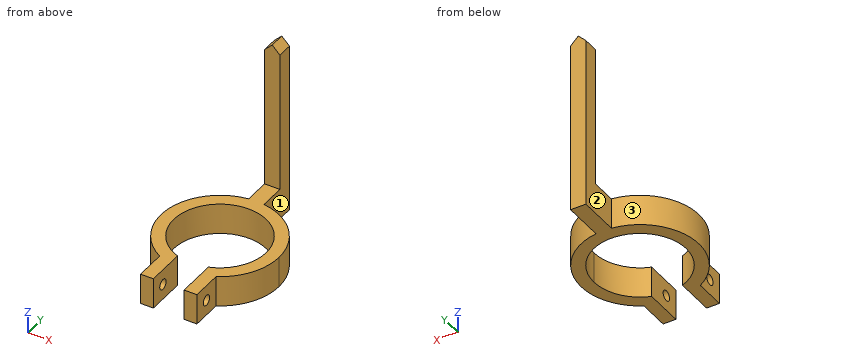
```python
from build123d import *

# Parameters (mm, degrees)
F1_DEPTH = 6
F2_W     = 3
F2_H     = 3
F3_DEPTH = 29
F5_D     = 2
F6_SIZE  = 1.49999


# Not quite as in the source:
# - a fillet or chamfer is up to 0.001 mm smaller than in the source, because OpenCascade refuses the exact size


with BuildPart() as f1:
    # F0 (on Top) → F1 (new body)
    with BuildSketch(Plane.XY):
        with BuildLine():
            ThreePointArc((-3, -8.4852813742), (-5.1961524227, 7.3484692283), (9, 0))
            ThreePointArc((9, 0), (7.3484692283, -5.1961524227), (3, -8.4852813742))
            Line((3, -8.4852813742), (3, -11.1018016556))
            ThreePointArc((3, -11.1018016556), (4.2794450198, -10.6740971666), (5.5, -10.0995049384))
            ThreePointArc((5.5, -10.0995049384), (9.8868599666, -5.8736700622), (11.5, 0))
            ThreePointArc((11.5, 0), (8.6458082329, 7.5828754441), (1.5, 11.401754251))
            ThreePointArc((1.5, 11.401754251), (0, 11.5), (-1.5, 11.401754251))
            ThreePointArc((-1.5, 11.401754251), (-11.3060177199, 2.103321972), (-5.5, -10.0995049384))
            ThreePointArc((-5.5, -10.0995049384), (-4.2794450198, -10.6740971666), (-3, -11.1018016556))
            Line((-3, -11.1018016556), (-3, -8.4852813742))
        make_face()
        with BuildLine():
            ThreePointArc((5.5, -10.0995049384), (4.2794450198, -10.6740971666), (3, -11.1018016556))
            Line((3, -11.1018016556), (3, -16.0995049384))
            Line((3, -16.0995049384), (5.5, -16.0995049384))
            Line((5.5, -16.0995049384), (5.5, -10.0995049384))
        make_face()
        with BuildLine():
            Line((-3, -16.0995049384), (-3, -11.1018016556))
            ThreePointArc((-3, -11.1018016556), (-4.2794450198, -10.6740971666), (-5.5, -10.0995049384))
            Line((-5.5, -10.0995049384), (-5.5, -16.0995049384))
            Line((-5.5, -16.0995049384), (-3, -16.0995049384))
        make_face()
        with BuildLine():
            Line((-1.5, 19.401754251), (-1.5, 11.401754251))
            ThreePointArc((-1.5, 11.401754251), (0, 11.5), (1.5, 11.401754251))
            Line((1.5, 11.401754251), (1.5, 19.401754251))
            Line((1.5, 19.401754251), (-1.5, 19.401754251))
        make_face()
    extrude(amount=F1_DEPTH)

    # F2 (on face) → F3 (join)
    with BuildSketch(Plane.XY.offset(6)):
        with Locations((0, 17.901754251)):
            Rectangle(F2_W, F2_H)
    extrude(amount=F3_DEPTH)

    # F5 (through all)
    with Locations(Plane(origin=(-5.5, 0, 0), x_dir=(0, -1, 0), z_dir=(-1, 0, 0))):
        with Locations((13.0995049384, 3)):
            Hole(F5_D / 2)

    # F6 (size 1.5 in the source; OpenCascade refuses exactly that, so slightly less here)
    f6_edges = [f1.edges().sort_by_distance(p)[0] for p in [
        (1.5, 17.901754, 35),
        (-1.5, 17.901754, 35),
    ]]
    chamfer(f6_edges, length=F6_SIZE)


solid = f1.part
```
The model under review builds one solid part; all positions refer to its coordinate system, in mm. Face numbers are marked on the shaded views. A direction names the side the tool comes from. Round coordinates to 2 decimals unless told otherwise and drop trailing zeros. Write each loop counter-clockwise with the first axis right and the second up, starting at its lowest first coordinate (ties: lowest second). Pieces come first, ordered by that corner, then holes.
(1) We need section A-A on z = 3. Give the boundary of the cut face in (x, y).
(2) Machinability: for the marked faces 1, 2 and 3, which of the approach directions +Z, -Z, +X, -X, +Y, -Y give a long, thin tool a straight path to every point of the face, cutting with its end or side? Answer none if there is none.
(3) We need section C-C on y = 2. Give the boundary of the cut face in (x, z).
(4) Insertion check: pin 1 (8 mm diameter, centred on x = -4.5, y = -10.5, fed in from -Z); pin 2 (6.5 mm diameter, centred on y = -12.5, z = 4, fed in from -X); pin 3 (10 mm diameter, centred on y = 14.5, z = 25.5, fed in from -X); pin 4 (2 mm diameter, centred on y = 16, z = 18.5, fed in from +X). Each pin has a flat end and moves straight along its axis. Give the tip position at first contact, or say it passes through.
(5) We need section B-B on x = 8.5. Give the boundary of the cut face in (y, z).
(6) Wall thickness on L1, parallel to Z at x = 9.75, y = 3.5; L2, parallel to Y at x = 0, z = 1.55; L3, parallel to X at y = 17.5, z = 18.5: over which ranges is each line inside the solid? List them lowest first.
Findings below:
1. outline: (-5.5, -16.1) - (-3, -16.1) - (-3, -14.1) - (-5.5, -14.1) - close; (-5.5, -12.1) - (-3, -12.1) - (-3, -8.49) arc R9 cw (long way) to (3, -8.49) - (3, -12.1) - (5.5, -12.1) - (5.5, -10.1) arc R11.5 ccw to (1.5, 11.4) - (1.5, 19.4) - (-1.5, 19.4) - (-1.5, 11.4) arc R11.5 ccw to (-5.5, -10.1) - close; (3, -16.1) - (5.5, -16.1) - (5.5, -14.1) - (3, -14.1) - close
2. face 1: +Z, -Z, +X, +Y
2. face 2: +Z, -Z, -X, +Y
2. face 3: +Z, -Z, -X
3. outline: (-11.32, 0) - (-8.77, 0) - (-8.77, 6) - (-11.32, 6) - close; (8.77, 0) - (11.32, 0) - (11.32, 6) - (8.77, 6) - close
4. pin 1: stops at z = 0
4. pin 2: stops at x = -6.83
4. pin 3: stops at x = -1.5
4. pin 4: stops at x = 1.5
5. outline: (-7.75, 0) - (-2.96, 0) - (-2.96, 6) - (-7.75, 6) - close; (2.96, 0) - (7.75, 0) - (7.75, 6) - (2.96, 6) - close
6. L1: z = 0 to 6
6. L2: y = 9 to 19.4
6. L3: x = -1.5 to 1.5
